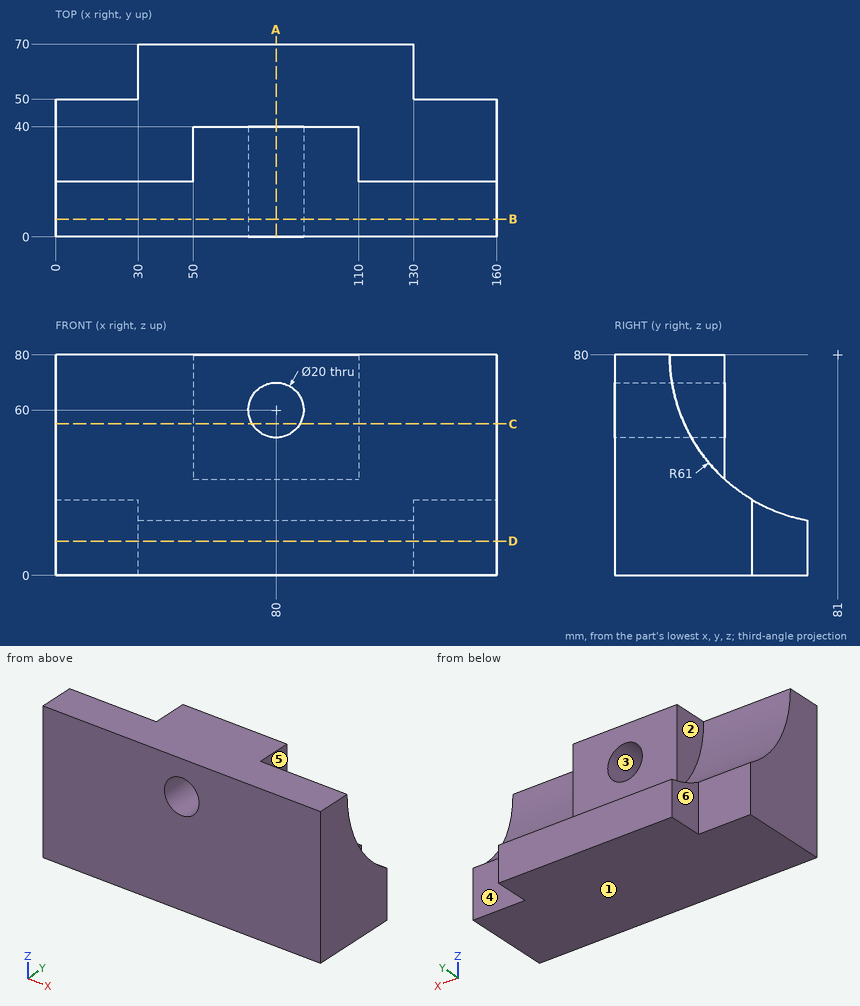
Can you work these out from the drawing? Everything is in mm from the part's minimum corner. A direction names the side the tool comes from. Coordinates: 2 decimals unless noted, no trailing zeros. Loops run counter-clockwise (first coordinate to the right, second up) from the corner with the lowest first, then second, coordinate; pieces in that order, holes last.
1. For P1, Ø18, axis at x = 80, z = 60, coming from the -Y side; P2, Ø1, axis at x = 31, z = 60.5, coming from the +Y side; P3, Ø16, axis at y = 61, z = 19.5, coming from the -X side; P4, Ø10, axis at y = 35, z = 53.5, coming from the -X side, each with a flat end and sliding along its axis, tell me the tip position at first contact or that it passes through.
2. For the marked faces 4, 5 and 6, which set-ups out of +Z, -Z, +X, -X, +Y, -Y let a thin tool reach every point of the face, with its end or its side?
3. Imagine slicing it at B-B, the plane y = 6.5. Please give me the cut outline in (x, z).
4. I need wall thicknesses on L1, parallel to X at y = 12, z = 60; L2, parallel to X at y = 26, z = 60; L3, parallel to Y at x = 91, z = 74. Which ranges of each line are inside material? Lowest first, please.
5. Imagine slicing it at A-A, the plane x = 80. Please give me the cut outline in (y, z), and give its area (3 significant figures).
6. Imagine slicing it at D-D, the plane z = 12.5. Please give me the cut outline in (x, y), and give its area (3 significant figures).
7. Imagine slicing it at C-C, the plane z = 55. Please give me the cut outline in (x, y), and give its area (3 significant figures).
8. If we mould it in two halves opening along X, with no side actions, what happens to the marked faces 1, 2 and 3? For each: pulls with the +X half, pulls with the -X half, needs draft (parallel to the pull), parting line crosses it, or undercut.
Taken from the geometry:
1. P1: passes through
1. P2: stops at y = 23.37
1. P3: stops at x = 30
1. P4: stops at x = 50
2. face 4: +Z, -Z, +X, +Y
2. face 5: +Z, +X, +Y
2. face 6: +Z, -Z, -X, +Y
3. outline: (0, 0) - (160, 0) - (160, 80) - (0, 80) - close; hole circle Ø20 at (80, 60)
4. L1: x = 0 to 70, 90 to 160
4. L2: x = 50 to 70, 90 to 110
4. L3: y = 0 to 40
5. outline: (0, 0) - (70, 0) - (70, 20) arc R61 cw to (40, 34.83) - (40, 50) - (0, 50) - close; (0, 70) - (40, 70) - (40, 80) - (0, 80) - close
5. area: 3,170 mm2
6. outline: (0, 0) - (160, 0) - (160, 50) - (130, 50) - (130, 70) - (30, 70) - (30, 50) - (0, 50) - close
6. area: 10,000 mm2
7. outline: (0, 0) - (71.34, 0) - (71.34, 40) - (50, 40) - (50, 25.36) - (0, 25.36) - close; (88.66, 0) - (160, 0) - (160, 25.36) - (110, 25.36) - (110, 40) - (88.66, 40) - close
7. area: 4,240 mm2
8. face 1: needs draft
8. face 2: pulls with the -X half
8. face 3: undercut
